For this review, take the finished solid that the model builds, in its own axes (mm). Coordinates: 2 decimals unless noted, no trailing zeros. Write each loop counter-clockwise with the first axis right and the second up, starting at its lowest first coordinate (ties: lowest second). Pieces come first, ordered by that corner, then holes. Notation, with made-up numbers: (66, 83) -> (89, 83) arc R25 ccw to (89, 108) -> close; hole circle Ø9 at (4.25, 30.25). An arc over 180 degrees is marked (long way). One line per item, written item: value. Start each with the question number.
1) For pin 1 Ø1.2 at (x, z) = (0, 1.25) entering from +Y, flat-tipped, find the tip position at first contact; note if it passes through.
2) For probe 1 along Z at (x, y) = (0, 0.7); probe 2 along Z at (x, y) = (-0.75, -0.45); probe 3 along X at (y, z) = (0.25, 22), list the stretches that pass through material, from the lowest coordinate up. Write a range as from..to.
3) Add section D-D (z = 17.5). State the section outline as (x, y) points.
4) Add section C-C (z = 41.75). State the section outline as (x, y) points.
5) Mouldability with a two-part tool opening along X and no side actions: class faces 1 (the flat face through (-5.75, 0, 21)), 2 (the flat face through (5.75, 0, 3)), 3 (the cylindrical face through (0.217, 0.018, 0.274)) as released by +X, released by -X, zero draft, split by the parting line, or undercut.
6) Add section B-B (x = 0). State the section outline as (y, z) points, and give its area (3 significant figures).
7) Add section A-A (y = -0.1). State the section outline as (x, z) points.
from build123d import *

# Parameters (mm, degrees)
F0_W     = 11.5
F0_H     = 2.5
F1_DEPTH = 43
F2_R     = 1
F3_DEPTH = 25
F5_DEPTH = 25


with BuildPart() as f1:
    # F0 (on Top) → F1 (new body)
    with BuildSketch(Plane.XY):
        Rectangle(F0_W, F0_H)
    extrude(amount=F1_DEPTH)

    # F2 (on face) → F3 (cut)
    with BuildSketch(Plane(origin=(0, 1.25, 0), x_dir=(-1, 0, 0), z_dir=(0, 1, 0))):
        with Locations((0, 1.25)):
            Circle(F2_R)
        with Locations((0, 41.75)):
            Circle(F2_R)
    extrude(amount=-F3_DEPTH, mode=Mode.SUBTRACT)

    # F4 (on face) → F5 (cut)
    with BuildSketch(Plane(origin=(0, 1.25, 0), x_dir=(-1, 0, 0), z_dir=(0, 1, 0))):
        with BuildLine():
            Line((-5.75, 26.404966), (-5.75, 5.576983))
            ThreePointArc((-5.75, 5.576983), (-2.61855, 15.990974), (-5.75, 26.404966))
        make_face()
    extrude(amount=-F5_DEPTH, mode=Mode.SUBTRACT)


solid = f1.part
Numbers:
1. pin 1: through
2. probe 1: 0..0.25, 2.25..40.75, 42.75..43
2. probe 2: 0..0.59, 1.91..41.09, 42.41..43
2. probe 3: -5.75..3.6
3. outline: (-5.75, -1.25) -> (2.68, -1.25) -> (2.68, 1.25) -> (-5.75, 1.25) -> close
4. outline: (-5.75, -1.25) -> (-1, -1.25) -> (-1, 1.25) -> (-5.75, 1.25) -> close; (1, -1.25) -> (5.75, -1.25) -> (5.75, 1.25) -> (1, 1.25) -> close
5. face 1: released by -X
5. face 2: released by +X
5. face 3: undercut
6. outline: (-1.25, 0) -> (1.25, 0) -> (1.25, 0.25) -> (-1.25, 0.25) -> close; (-1.25, 2.25) -> (1.25, 2.25) -> (1.25, 40.75) -> (-1.25, 40.75) -> close; (-1.25, 42.75) -> (1.25, 42.75) -> (1.25, 43) -> (-1.25, 43) -> close
6. area: 97.5 mm²
7. outline: (-5.75, 0) -> (5.75, 0) -> (5.75, 5.58) arc R18.88 cw to (5.75, 26.4) -> (5.75, 43) -> (-5.75, 43) -> close; hole circle Ø2 at (0, 1.25); hole circle Ø2 at (0, 41.75)
